Study the drawing (mm; zero at the part's minimum x, y, z) and answer. Give positions to 0.01 mm unless a question says otherwise; leave off trailing zeros. Answer as CSV lines item,"result". Start each with the question number.
1. A flat-ended cylindrical pin translates along its axis: pin 1 (1 mm diameter, centred on x = 5.5, z = 1, fed in from -Y). Find the tip coordinate at first contact, or state that the pin passes through.
2. Find the intervals of material crossed by L1, parallel to Y at x = 4.25, z = 1.55 (1 decimal); L2, parallel to Y at x = 5, z = 2.4 (1 decimal); L3, parallel to Y at x = 1.25, z = 1.65 (1 decimal), in increasing order.
3. A cutting plane is placed at A-A (z = 0.6). State how many separate pieces and enclosed holes the cut face has, then the cut area to 3 significant figures.
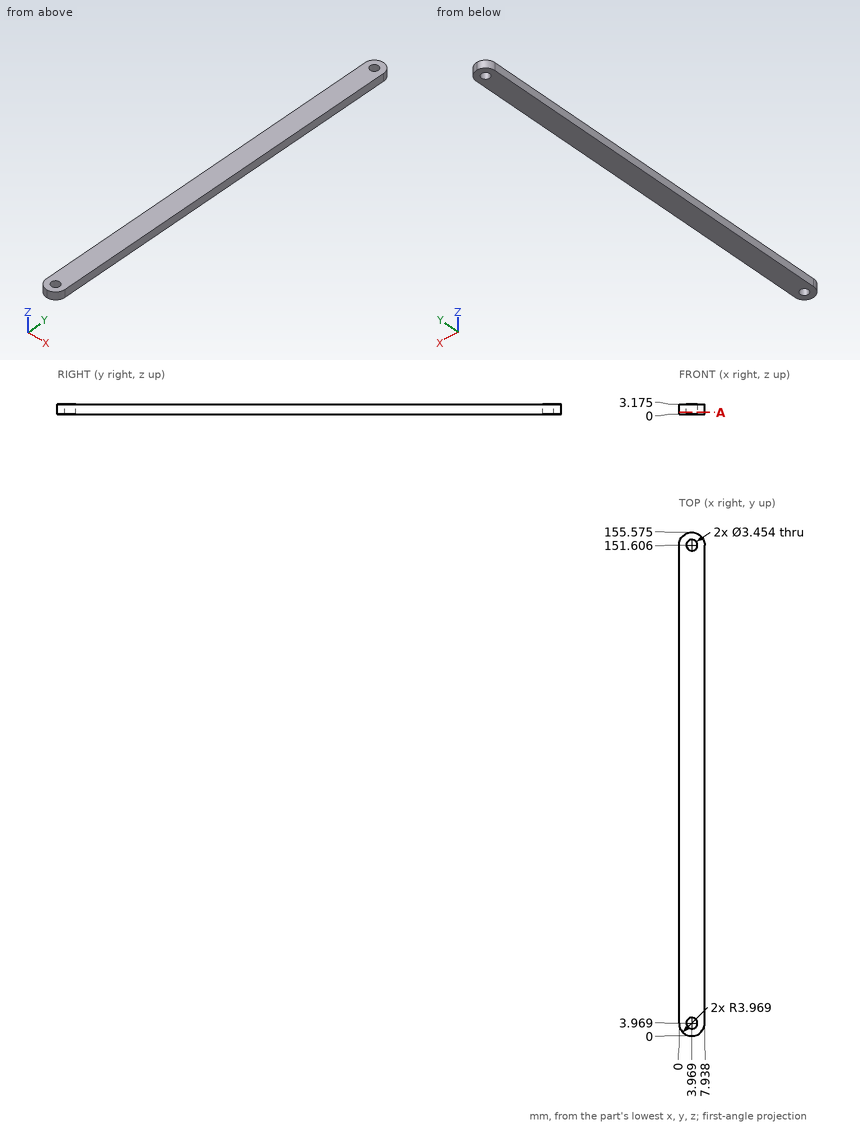
Answer sheet:
1,pin 1,"stops at y = 0.14"
2,L1,"y = 0 to 2.3, 5.7 to 149.9, 153.3 to 155.6"
2,L2,"y = 0.1 to 2.6, 5.4 to 150.2, 153 to 155.4"
2,L3,"y = 1.1 to 154.5"
3,separate pieces,"1"
3,enclosed holes,"2"
3,area,"1,200 mm^2"
